Can you work these out from the model? Positions are in its coordinate system, mm. Face numbers are marked on the shaded views. Coordinates: 2 decimals unless noted, no trailing zeros. Order: outer loops, then holes, each group sorted by start corner. A loop starts at its lowest first (then second) coordinate and runs counter-clockwise, first axis right, second up. Notation, with made-up numbers: (-9, 14) -> (49, 14) arc R21 ccw to (49, 40) -> close; hole circle Ø3 at (80, -39.75). An arc over 180 degrees is marked (long way). Return JSON: item names as keys, results as strings. Group by question number.
1) Thinking about a two-plate mould opening in X: for the marked faces 1, 2 and 3, which applies, +X half, -X half, draft (parallel to the pull), parting line (faces both ways), or undercut?
2) If we section it at B-B, the plane y = -15: Please give me the cut outline in (x, z) (3 decimals).
3) If we section it at A-A, the plane z = -25.4: Please give me the cut outline in (x, y).
4) For pin 1 (1.5 mm diameter, centred on x = 14.5, z = -33.5, fed in from +Y), with a flat end and sliding along its axis, tell me the tip position at first contact or that it passes through.
5) If we section it at D-D, the plane y = -22.5: Please give me the cut outline in (x, z) (3 decimals), then the cut area to 3 significant figures.
6) If I drill on probe 1 along Z at (x, y) = (31, -14.75); probe 2 along X at (y, z) = (-17.5, -14.5); probe 3 along Z at (x, y) = (36.5, -3.25), over which ranges is the centre line in solid material (lowest first)? Write a range as from..to.
7) If we section it at C-C, the plane x = 6: Please give me the cut outline in (y, z), then the cut area to 3 significant figures.
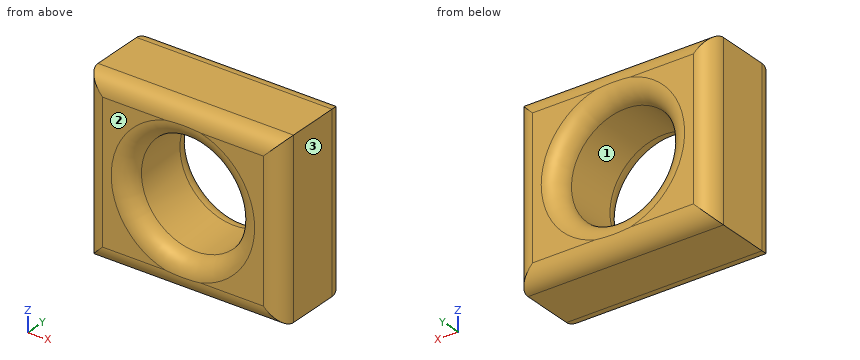
from build123d import *

# Parameters (mm, degrees)
F0_W        = 57.15
F0_H        = 50.8
F1_DEPTH    = 25.4
F2_DEPTH    = 25.4
F3_DEPTH    = 25.4
F4_R        = 15.875
F5_DEPTH    = 25.4
F6_T1_DEPTH = 82.55
F6_T3_DEPTH = 76.2
F7_T1_DEPTH = 82.55
F7_T3_DEPTH = 76.2


# Not quite as in the source:
# - a fillet or chamfer that OpenCascade refuses, or shapes differently, is made with other operations: its cross-section is extruded or revolved along the edge and cut away or added


with BuildPart() as f1:
    # F0 (on Front) → F1 (new body)
    with BuildSketch(Plane.XZ):
        with Locations((28.575, -25.4)):
            Rectangle(F0_W, F0_H)
    extrude(amount=F1_DEPTH)

    # F0 (on Front) → F2 (join)
    with BuildSketch(Plane.XZ):
        with Locations((28.575, -25.4)):
            Rectangle(F0_W, F0_H)
    extrude(amount=F2_DEPTH)

    # F0 (on Front) → F3 (join)
    with BuildSketch(Plane.XZ):
        with Locations((28.575, -25.4)):
            Rectangle(F0_W, F0_H)
    extrude(amount=F3_DEPTH)

    # F4 (on face) → F5 (cut)
    with BuildSketch(Plane.XZ.offset(25.4)):
        with Locations((28.575, -25.4)):
            Circle(F4_R)
    extrude(amount=-F5_DEPTH, mode=Mode.SUBTRACT)

    # F6: fillet of radius 5.08 on 5 edges, made by hand

    # F6_s2 → F6_t1 (cut)
    with BuildSketch(Plane.YZ.offset(-12.7)):
        with BuildLine():
            ThreePointArc((-20.32, 0), (-23.9121024484, -1.4878975516), (-25.4, -5.08))
            Line((-25.4, -5.08), (-25.4, 0))
            Line((-25.4, 0), (-20.32, 0))
        make_face()
        with BuildLine():
            ThreePointArc((-25.4, -45.72), (-23.9121024484, -49.3121024484), (-20.32, -50.8))
            Line((-20.32, -50.8), (-25.4, -50.8))
            Line((-25.4, -50.8), (-25.4, -45.72))
        make_face()
    extrude(amount=F6_T1_DEPTH, mode=Mode.SUBTRACT)

    # F6_s4 → F6_t3 (cut)
    with BuildSketch(Plane.XY.offset(-63.5)):
        with BuildLine():
            ThreePointArc((57.15, -20.32), (55.6621024484, -23.9121024484), (52.07, -25.4))
            Line((52.07, -25.4), (57.15, -25.4))
            Line((57.15, -25.4), (57.15, -20.32))
        make_face()
        with BuildLine():
            ThreePointArc((0, -20.32), (1.4878975516, -23.9121024484), (5.08, -25.4))
            Line((5.08, -25.4), (0, -25.4))
            Line((0, -25.4), (0, -20.32))
        make_face()
    extrude(amount=F6_T3_DEPTH, mode=Mode.SUBTRACT)

    # F6_s5 → F6_t6 (revolve, cut)
    with BuildSketch(Plane.XY.offset(-25.4)):
        with BuildLine():
            ThreePointArc((49.53, -25.4), (45.9378975516, -23.9121024484), (44.45, -20.32))
            Line((44.45, -20.32), (44.45, -25.4))
            Line((44.45, -25.4), (49.53, -25.4))
        make_face()
    revolve(axis=Axis((28.575, -25.4, -25.4), (0, -1, 0)), mode=Mode.SUBTRACT)

    # F7: fillet of radius 5.08 on 5 edges, made by hand

    # F7_s2 → F7_t1 (cut)
    with BuildSketch(Plane.YZ.offset(-12.7)):
        with BuildLine():
            ThreePointArc((-5.08, 0), (-1.4878975516, -1.4878975516), (0, -5.08))
            Line((0, -5.08), (0, 0))
            Line((0, 0), (-5.08, 0))
        make_face()
        with BuildLine():
            ThreePointArc((0, -45.72), (-1.4878975516, -49.3121024484), (-5.08, -50.8))
            Line((-5.08, -50.8), (0, -50.8))
            Line((0, -50.8), (0, -45.72))
        make_face()
    extrude(amount=F7_T1_DEPTH, mode=Mode.SUBTRACT)

    # F7_s4 → F7_t3 (cut)
    with BuildSketch(Plane.XY.offset(-63.5)):
        with BuildLine():
            ThreePointArc((52.07, 0), (55.6621024484, -1.4878975516), (57.15, -5.08))
            Line((57.15, -5.08), (57.15, 0))
            Line((57.15, 0), (52.07, 0))
        make_face()
        with BuildLine():
            ThreePointArc((5.08, 0), (1.4878975516, -1.4878975516), (0, -5.08))
            Line((0, -5.08), (0, 0))
            Line((0, 0), (5.08, 0))
        make_face()
    extrude(amount=F7_T3_DEPTH, mode=Mode.SUBTRACT)

    # F7_s5 → F7_t6 (revolve, cut)
    with BuildSketch(Plane.XY.offset(-25.4)):
        with BuildLine():
            ThreePointArc((49.53, 0), (45.9378975516, -1.4878975516), (44.45, -5.08))
            Line((44.45, -5.08), (44.45, 0))
            Line((44.45, 0), (49.53, 0))
        make_face()
    revolve(axis=Axis((28.575, 0, -25.4), (0, -1, 0)), mode=Mode.SUBTRACT)


solid = f1.part
Result sheet:
{
 "1": {"face 1": "undercut", "face 2": "draft", "face 3": "+X half"},
 "2": {"outline": "(0, -50.8) -> (57.15, -50.8) -> (57.15, 0) -> (0, 0) -> close; hole circle Ø31.75 at (28.575, -25.4)"},
 "3": {"outline": "(0, -20.32) arc R5.08 ccw to (5.08, -25.4) -> (7.62, -25.4) arc R5.08 ccw to (12.7, -20.32) -> (12.7, -5.08) arc R5.08 ccw to (7.62, 0) -> (5.08, 0) arc R5.08 ccw to (0, -5.08) -> close; (44.45, -20.32) arc R5.08 ccw to (49.53, -25.4) -> (52.07, -25.4) arc R5.08 ccw to (57.15, -20.32) -> (57.15, -5.08) arc R5.08 ccw to (52.07, 0) -> (49.53, 0) arc R5.08 ccw to (44.45, -5.08) -> close"},
 "4": {"pin 1": "stops at y = -1.91"},
 "5": {"outline": "(0.492, -50.308) -> (56.658, -50.308) -> (56.658, -0.492) -> (0.492, -0.492) -> close; hole circle Ø32.733 at (28.575, -25.4)", "area": "1,960 mm2"},
 "6": {"probe 1": "z = -50.8..-41.09, -9.71..0", "probe 2": "x = 0..17.03, 40.12..57.15", "probe 3": "z = -50.46..-39.55, -11.25..-0.34"},
 "7": {"outline": "(-25.4, -45.72) arc R5.08 ccw to (-20.32, -50.8) -> (-5.08, -50.8) arc R5.08 ccw to (0, -45.72) -> (0, -5.08) arc R5.08 ccw to (-5.08, 0) -> (-20.32, 0) arc R5.08 ccw to (-25.4, -5.08) -> close", "area": "1,270 mm2"}
}
